For this review, take the finished solid that the model builds, in its own axes (mm). Face numbers are marked on the shaded views. A direction names the side the tool comes from. Give positions to 0.01 mm unless a question says otherwise; leave off trailing zeros. Write each loop counter-clockwise with the first axis right and the second up, starting at its lowest first coordinate (ties: lowest second). Pieces come first, ordered by that corner, then holes.
1) We need section D-D on z = 3.5. Give the boundary of the cut face in (x, y), and give its area (3 significant figures).
2) Wall thickness on line 1 along Z through (x, y) = (0, -0.75); line 2 along X through (y, z) = (-1.25, 10.75); line 3 along Y through (x, z) = (1, 13.25): over which ranges is each line inside the solid? List them lowest first.
3) We need section C-C on z = 13.5. Give the boundary of the cut face in (x, y), and give its area (3 significant figures).
4) We need section A-A on y = 0. Give the boundary of the cut face in (x, z).
5) Machinability: for the marked faces 5, 6, 7, 8 and 9, which of the approach directions +Z, -Z, +X, -X, +Y, -Y give a long, thin tool a straight path to every point of the face, cutting with its end or side? Answer none if there is none.
6) For P1, Ø3, axis at y = 0.5, z = 12.5, coming from the +X side; P2, Ø4, axis at x = -4.5, y = 2, coming from the +Z side; P3, Ø2, axis at x = -3, z = 6.5, coming from the -Y side, all flat-tipped, find the tip position at first contact; note any pin that passes through.
7) We need section B-B on x = 0. Give the number of separate pieces and of enclosed holes in the cut face, and give its area (3 significant figures).
8) Draft analysis for pull direction Z (two halves, no side actions). For the marked faces 1, 2, 3 and 4, state which applies: pulls with the +Z half, pulls with the -Z half, needs draft (parallel to the pull), parting line crosses it, or undercut.
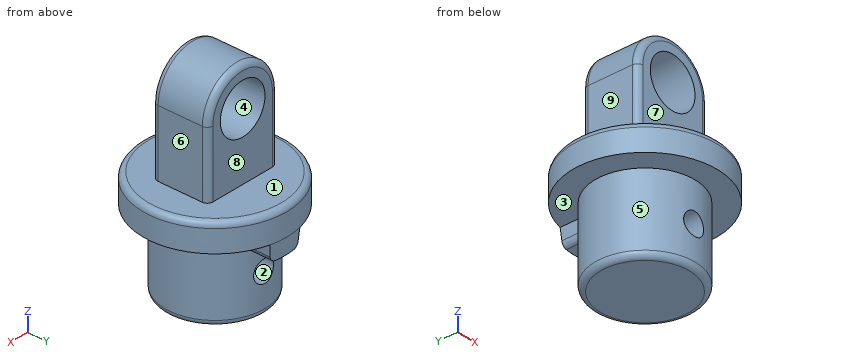
from build123d import *

# Parameters (mm, degrees)
ESQUISSE1_R             = 4.5
BASE_EXTRUSION_DEPTH    = 7
ESQUISSE2_R             = 6.5
BOSS_EXTRU_1_DEPTH      = 2.5
BOSS_EXTRU_2_DEPTH      = 2.5
ESQUISSE4_R             = 2.25
ESQUISSE4_R_2           = 1
ENL_V_MAT_EXTRU_1_DEPTH = 22.5
BOSS_EXTRU_3_DEPTH      = 1.5
BOSS_EXTRU_3_TAPER      = 5
CONG_1_R                = 0.5


with BuildPart() as part:
    # Esquisse1 → Base-Extrusion (new body)
    with BuildSketch(Plane.XY):
        Circle(ESQUISSE1_R)
    extrude(amount=BASE_EXTRUSION_DEPTH)

    # Esquisse2 → Boss.-Extru.1 (add)
    with BuildSketch(Plane.XY.offset(7)):
        Circle(ESQUISSE2_R)
    extrude(amount=BOSS_EXTRU_1_DEPTH)

    # Esquisse3 → Boss.-Extru.2 (add, symmetric)
    with BuildSketch(Plane(origin=(0, 0, 0), x_dir=(1, 0, 0), z_dir=(0, 1, 0))):
        with BuildLine():
            Line((-3.5, -9.5), (-3.5, -15.5))
            ThreePointArc((-3.5, -15.5), (0, -19), (3.5, -15.5))
            Line((3.5, -15.5), (3.5, -9.5))
            Line((3.5, -9.5), (-3.5, -9.5))
        make_face()
    extrude(amount=BOSS_EXTRU_2_DEPTH, both=True)

    # Esquisse4 → Enlèv. mat.-Extru.1 (cut, symmetric)
    with BuildSketch(Plane(origin=(0, 2.5, 0), x_dir=(-1, 0, 0), z_dir=(0, 1, 0))):
        with Locations((0, 15.5)):
            Circle(ESQUISSE4_R)
        with Locations((0, 3.5)):
            Circle(ESQUISSE4_R_2)
    extrude(amount=ENL_V_MAT_EXTRU_1_DEPTH, both=True, mode=Mode.SUBTRACT)

    # Esquisse5 → Boss.-Extru.3 (add)
    with BuildSketch(Plane(origin=(0, 0, 7), x_dir=(-1, 0, 0), z_dir=(0, 0, -1))):
        with BuildLine():
            ThreePointArc((1.5, 6.32455532), (0, 6.5), (-1.5, 6.32455532))
            Line((-1.5, 6.32455532), (-1.5, 4))
            Line((-1.5, 4), (1.5, 4))
            Line((1.5, 4), (1.5, 6.32455532))
        make_face()
    extrude(amount=BOSS_EXTRU_3_DEPTH, taper=BOSS_EXTRU_3_TAPER)

    # Congé1
    cong_1_edges = [part.edges().sort_by_distance(p)[0] for p in [
        (-6.5, 0, 9.5),
        (-1.368767005, 5.253360318, 5.5),
        (-4.5, 0, 0),
        (1.368767005, 5.253360318, 5.5),
        (-3.5, -2.5, 12.5),
        (-3.5, 2.5, 12.5),
        (0, -2.5, 19),
        (3.5, -2.5, 12.5),
        (3.5, 2.5, 12.5),
        (0, 2.5, 19),
    ]]
    fillet(cong_1_edges, radius=CONG_1_R)


solid = part.part
Results list:
1. outline: (-1, -4.39) - (-1, 4.39) arc R4.5 ccw to start; (1, -4.39) arc R4.5 ccw to (1, 4.39) - close
1. area: 45.8 mm2
2. line 1: z = 0 to 2.5, 4.5 to 13.25, 17.75 to 19
2. line 2: x = -3.5 to 3.5
2. line 3: y = -2.5 to 2.5
3. outline: (-3.5, -2) arc R0.5 ccw to (-3, -2.5) - (-1.03, -2.5) - (-1.03, 2.5) - (-3, 2.5) arc R0.5 ccw to (-3.5, 2) - close; (1.03, -2.5) - (3, -2.5) arc R0.5 ccw to (3.5, -2) - (3.5, 2) arc R0.5 ccw to (3, 2.5) - (1.03, 2.5) - close
3. area: 24.5 mm2
4. outline: (-6.5, 7) - (-4.5, 7) - (-4.5, 0.5) arc R0.5 ccw to (-4, 0) - (4, 0) arc R0.5 ccw to (4.5, 0.5) - (4.5, 7) - (6.5, 7) - (6.5, 9) arc R0.5 ccw to (6, 9.5) - (3.5, 9.5) - (3.5, 15.5) arc R3.5 ccw to (-3.5, 15.5) - (-3.5, 9.5) - (-6, 9.5) arc R0.5 ccw to (-6.5, 9) - close; hole circle Ø4.5 at (0, 15.5); hole circle Ø2 at (0, 3.5)
5. face 5: -Z
5. face 6: +Z, +X, +Y, -Y
5. face 7: +Z, +X, -X, -Y
5. face 8: +Z, +X, -X, +Y
5. face 9: +Z, -X, +Y, -Y
6. P1: stops at x = 3.5
6. P2: stops at z = 17.95
6. P3: stops at y = -6.14
7. separate pieces: 3
7. enclosed holes: 0
7. area: 105 mm2
8. face 1: pulls with the +Z half
8. face 2: undercut
8. face 3: pulls with the -Z half
8. face 4: undercut
